```python
from build123d import *

# Parameters (mm, degrees)
BOSS_EXTRUDE1_DEPTH = 3
SKETCH2_R           = 1.5
CUT_EXTRUDE1_DEPTH  = 10


with BuildPart() as part:
    # Sketch1 → Boss-Extrude1 (new body)
    with BuildSketch(Plane.XY):
        with BuildLine():
            Line((0, 0), (-97.320508076, 0))
            ThreePointArc((-97.320508076, 0), (-99.908698527, -0.340741737), (-102.320508076, -1.339745962))
            Line((-102.320508076, -1.339745962), (-147.834936491, -27.617513459))
            ThreePointArc((-147.834936491, -27.617513459), (-148.999751056, -29.135529356), (-148.75, -31.032576969))
            Line((-148.75, -31.032576969), (-146.364135626, -35.165015284))
            ThreePointArc((-146.364135626, -35.165015284), (-144.740171152, -36.355755302), (-142.765131026, -35.962895395))
            Line((-142.765131026, -35.962895395), (-108.249632243, -11.794882962))
            ThreePointArc((-108.249632243, -11.794882962), (-108.142543563, -11.71556254), (-108.039833804, -11.630648348))
            ThreePointArc((-108.039833804, -11.630648348), (-87.659186574, -4.241562471), (-67.620976195, -12.514379188))
            ThreePointArc((-67.620976195, -12.514379188), (-64.029298108, -14.71197301), (-59.851424349, -15.236321126))
            Line((-59.851424349, -15.236321126), (0, -10))
            Line((0, -10), (0, 0))
        make_face()
    extrude(amount=BOSS_EXTRUDE1_DEPTH)

    # Sketch2 → Cut-Extrude1 (cut)
    with BuildSketch(Plane(origin=(0, 0, 0), x_dir=(-1, 0, 0), z_dir=(0, 0, -1))):
        with Locations((5, -5)):
            Circle(SKETCH2_R)
        with Locations((62, -5)):
            Circle(SKETCH2_R)
    extrude(amount=-CUT_EXTRUDE1_DEPTH, mode=Mode.SUBTRACT)


solid = part.part
```
The listing builds one solid part. Answer for the finished solid, in the listing's coordinates (mm). Round coordinates to 2 decimals unless told otherwise and drop trailing zeros. Order: outer loops, then holes, each group sorted by start corner. A loop starts at its lowest first (then second) coordinate and runs counter-clockwise, first axis right, second up. Notation, with made-up numbers: (89, -18) - (103, -18) arc R11 ccw to (103, -5) - close; hole circle Ø4 at (-27, 11.5). An arc over 180 degrees is marked (long way). Put each result on its own line as item: value. Start each with the question number.
(1) Find section A-A (z = 1.25). Give the vertices of the cut face in (x, y), plus the area to 3 significant figures.
(2) Find section D-D (x = -128). Give the vertices of the cut face in (y, z), plus the area to 3 significant figures.
(3) Find section C-C (x = -62). Give the vertices of the cut face in (y, z).
(4) Straight lines are drawn through the part: probe 1 along Y at (x, z) = (-5, 2.45); probe 2 along Y at (x, z) = (-62, 1.95); probe 3 along X at (y, z) = (-34, 2.05). For each, find the intervals that lie inside material, in ascending order. Write a range as from..to.
(5) Find section B-B (y = -14). Give the vertices of the cut face in (x, z), plus the area to 3 significant figures.
(6) Determine the mould class of faces 1 (the cylindrical face through (-63.43, -4.55, 1.48)), 2 (the cylindrical face through (-99.87, -0.33, 1.48)), 3 (the cylindrical face through (-144.77, -36.35, 1.48)) for opening direction X: released by +X, released by -X, zero draft, split by the parting line, or undercut.
(7) Given P1, Ø1.5, axis at y = -6.5, z = 2.5, coming from the -X side; P2, Ø1.5, axis at x = -36.5, z = 2, coming from the -Y side; P3, Ø1.5, axis at x = -62, z = 2, coming from the -Y side, each flat-ended and moving along its own axis, determine where each tip first touches the part or whether it passes through.
Reply:
1. outline: (-148.75, -31.03) - (-146.36, -35.17) arc R2.5 ccw to (-142.77, -35.96) - (-108.25, -11.79) arc R2.5 ccw to (-108.04, -11.63) arc R30 cw to (-67.62, -12.51) arc R10 ccw to (-59.85, -15.24) - (0, -10) - (0, 0) - (-97.32, 0) arc R10 ccw to (-102.32, -1.34) - (-147.83, -27.62) arc R2.5 ccw to start; hole circle Ø3 at (-62, -5); hole circle Ø3 at (-5, -5)
1. area: 1,470 mm^2
2. outline: (-25.62, 0) - (-16.17, 0) - (-16.17, 3) - (-25.62, 3) - close
2. area: 28.4 mm^2
3. outline: (-15.19, 0) - (-6.5, 0) - (-6.5, 3) - (-15.19, 3) - close; (-3.5, 0) - (0, 0) - (0, 3) - (-3.5, 3) - close
4. probe 1: -10.44..-6.5, -3.5..0
4. probe 2: -15.19..-6.5, -3.5..0
4. probe 3: -147.04..-139.96
5. outline: (-124.25, 0) - (-111.4, 0) - (-111.4, 3) - (-124.25, 3) - close; (-65.61, 0) - (-45.72, 0) - (-45.72, 3) - (-65.61, 3) - close
5. area: 98.2 mm^2
6. face 1: undercut
6. face 2: released by -X
6. face 3: split by the parting line
7. P1: x = -112.56
7. P2: y = -13.26
7. P3: y = -15.26
